from build123d import *

# Parameters (mm, degrees)
BOSS_EXTRUDE1_DEPTH = 2
BOSS_EXTRUDE2_DEPTH = 2
BOSS_EXTRUDE3_DEPTH = 2


with BuildPart() as part:
    # Sketch1 → Boss-Extrude1 (new body)
    with BuildSketch(Plane(origin=(0, 0, 0), x_dir=(1, 0, 0), z_dir=(0, 1, 0))):
        Polygon((-232.5, 215), (-222.5, 225), (222.5, 225), (232.5, 215), (232.5, -215), (222.5, -225), (-222.5, -225), (-232.5, -215), align=None)
    extrude(amount=BOSS_EXTRUDE1_DEPTH)

    # Sketch3 → Boss-Extrude2 (add)
    with BuildSketch(Plane.XY.offset(225)):
        Polygon((-222.5, 2), (222.5, 2), (196.5, 32), (-196.5, 32), align=None)
    boss_extrude2 = extrude(amount=-BOSS_EXTRUDE2_DEPTH)

    # Sketch4 → Boss-Extrude3 (add)
    with BuildSketch(Plane.ZY.offset(232.5)):
        Polygon((-215, 2), (215, 2), (190, 32), (-190, 32), align=None)
    boss_extrude3 = extrude(amount=-BOSS_EXTRUDE3_DEPTH)

    # Mirror2: Boss-Extrude3 across plane
    add(boss_extrude3.mirror(Plane(origin=(0, 0, 0), x_dir=(0, 0, 1), z_dir=(1, 0, 0))))

    # Mirror3: Boss-Extrude2 across plane
    add(boss_extrude2.mirror(Plane.XY))


solid = part.part
Geometry: final body of the model. Coordinates: model frame, mm. A direction names the side the tool comes from. Coordinates: 2 decimals unless noted, no trailing zeros. Loops run counter-clockwise (first coordinate to the right, second up) from the corner with the lowest first, then second, coordinate; pieces in that order, holes last. Notation, with made-up numbers: (34.25, 70.5) - (60.25, 70.5) arc R36 cw to (60.25, 108.5) - close; hole circle Ø6 at (56, 65). An arc over 180 degrees is marked (long way). Put each result on its own line as item: value. Start each with the question number.
Q1. Cut plane A-A, the plane y = 24.5. Return loops of the section in (x, z).
Q2. Cut plane B-B, the plane x = 24. Return loops of the section in (y, z), and give its area (3 significant figures).
Q3. Pull-direction query (Z, two-part tool) for faces 4 (the flat face through (3, 2, -3)), 5 (the flat face through (230.5, 17, -3)), 6 (the flat face through (227.6, 1, 219.9)); classes: released by +Z, released by -Z, zero draft, split by the parting line, or undercut.
Q4. Cut plane C-C, the plane z = -196.5. Return loops of the section in (x, y), and give its area (3 significant figures).
Q5. Line query: line 1 (X direction, y = 14.5, z = -56.5); line 2 (Z direction, x = -136, y = 7.5); line 3 (Y direction, x = -175, z = -73). Output: solid intervals per line, ascending.
Q6. Set-up query: faces 1 (the flat face through (-230.5, 17, -3)), 2 (the flat face through (-3, 17, 223)), 3 (the flat face through (231.514, 16.79, 202.675)). Return all of +Z, -Z, +X, -X, +Y, -Y with unobstructed straight access to the full face (end or side cutting, diameter ignored); none if empty.
Filled sheet:
1. outline: (-232.5, -196.25) - (-230.5, -196.25) - (-230.5, 196.25) - (-232.5, 196.25) - close; (-203, -225) - (203, -225) - (203, -223) - (-203, -223) - close; (-203, 223) - (203, 223) - (203, 225) - (-203, 225) - close; (230.5, -196.25) - (232.5, -196.25) - (232.5, 196.25) - (230.5, 196.25) - close
2. outline: (0, -225) - (32, -225) - (32, -223) - (2, -223) - (2, 223) - (32, 223) - (32, 225) - (0, 225) - close
2. area: 1,020 mm²
3. face 4: undercut
3. face 5: zero draft
3. face 6: released by +Z
4. outline: (-232.5, 0) - (232.5, 0) - (232.5, 24.2) - (230.5, 24.2) - (230.5, 2) - (-230.5, 2) - (-230.5, 24.2) - (-232.5, 24.2) - close
4. area: 1,020 mm²
5. line 1: -232.5 to -230.5, 230.5 to 232.5
5. line 2: -225 to -223, 223 to 225
5. line 3: 0 to 2
6. face 1: +Z, -Z, +Y
6. face 2: +X, -X, +Y
6. face 3: +Z, +X, -X, +Y
